For this review, take the finished solid that the model builds, in its own axes (mm). Give positions to 0.01 mm unless a question says otherwise; leave off trailing zeros. Order: outer loops, then holes, each group sorted by start corner. A loop starts at its lowest first (then second) coordinate and runs counter-clockwise, first axis right, second up.
Item 1: Consider section A-A (x = 0). Give the boundary of the cut face in (y, z).
Item 2: For probe 1 along X at (y, z) = (-40.5, -74); probe 2 along Y at (x, z) = (0, -71.5); probe 3 along Y at (x, z) = (-16.15, -70.75), list the stretches that pass through material, from the lowest coordinate up.
Item 3: Consider section C-C (x = 18.5). Give the boundary of the cut face in (y, z).
Item 4: For P1, Ø9.5, axis at x = 37.5, y = 0, coming from the +Z side; P2, Ø2.5, axis at x = 57, y = 24.5, coming from the +Z side, all flat-tipped, find the tip position at first contact; note any pin that passes through.
Item 5: Consider section D-D (x = 44). Give the boundary of the cut face in (y, z).
Item 6: Consider section B-B (x = 58.85). Give the boundary of the cut face in (y, z), plus the area to 3 significant figures.
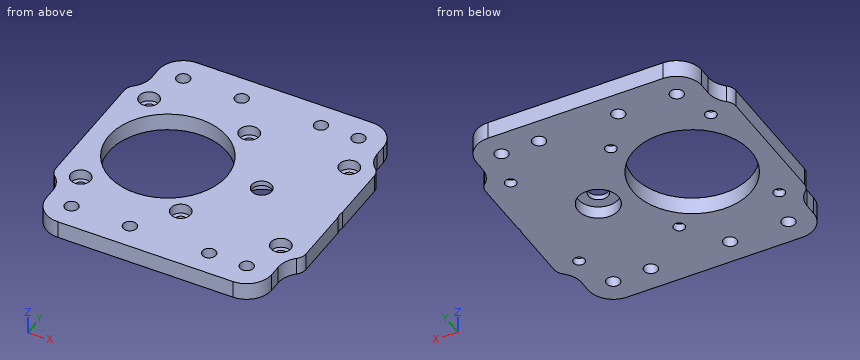
```python
from build123d import *

# Parameters (mm, degrees)
SKETCH2_R                      = 2.15
SKETCH2_R_2                    = 23.6
BOSS_EXTRUDE1_DEPTH            = 7
CUT_EXTRUDE1_START             = -7
SKETCH3_R                      = 8.1
SKETCH3_R_2                    = 23.6
CUT_EXTRUDE1_DEPTH             = 5
SKETCH4_R                      = 4
CUT_EXTRUDE2_DEPTH             = 5
SKETCH5_R                      = 6.365
CUT_EXTRUDE3_DEPTH             = 10
CBORE_FOR_M4_SHCS1_D           = 4.5
CBORE_FOR_M4_SHCS1_CBORE_D     = 8
CBORE_FOR_M4_SHCS1_CBORE_DEPTH = 4
SKETCH9_W                      = 90
SKETCH9_H                      = 20.85
SKETCH9_R                      = 2.7
BOSS_EXTRUDE3_DEPTH            = 7
FILLET2_R                      = 10
SKETCH10_W                     = 55
SKETCH10_H                     = 101.7
SKETCH10_R                     = 23.6
SKETCH10_R_2                   = 2.25
SKETCH10_R_3                   = 2.7
BOSS_EXTRUDE4_DEPTH            = 7


with BuildPart() as part:
    # Sketch2 → Boss-Extrude1 (new body)
    with BuildSketch(Plane.XY.offset(-75.526253649)):
        with BuildLine():
            Line((63.85, 30), (-26.15, 30))
            ThreePointArc((-26.15, 30), (-29.685533906, 28.535533906), (-31.15, 25))
            Line((-31.15, 25), (-31.15, -25))
            ThreePointArc((-31.15, -25), (-29.685533906, -28.535533906), (-26.15, -30))
            Line((-26.15, -30), (63.85, -30))
            ThreePointArc((63.85, -30), (67.385533906, -28.535533906), (68.85, -25))
            Line((68.85, -25), (68.85, 25))
            ThreePointArc((68.85, 25), (67.385533906, 28.535533906), (63.85, 30))
        make_face()
        with Locations((58.85, 25)):
            Circle(SKETCH2_R, mode=Mode.SUBTRACT)
        with Locations((18.85, 25)):
            Circle(SKETCH2_R, mode=Mode.SUBTRACT)
        with Locations((-21.15, 25)):
            Circle(SKETCH2_R, mode=Mode.SUBTRACT)
        with Locations((-21.15, -25)):
            Circle(SKETCH2_R, mode=Mode.SUBTRACT)
        with Locations((18.85, -25)):
            Circle(SKETCH2_R, mode=Mode.SUBTRACT)
        with Locations((58.85, -25)):
            Circle(SKETCH2_R, mode=Mode.SUBTRACT)
        Circle(SKETCH2_R_2, mode=Mode.SUBTRACT)
    extrude(amount=BOSS_EXTRUDE1_DEPTH)

    # Sketch3 → Cut-Extrude1 (cut)
    with BuildSketch(Plane.XY.offset(-68.526253649).offset(CUT_EXTRUDE1_START)):
        with Locations((37.5, 0)):
            Circle(SKETCH3_R)
        Circle(SKETCH3_R_2)
    extrude(amount=CUT_EXTRUDE1_DEPTH, mode=Mode.SUBTRACT)

    # Sketch4 → Cut-Extrude2 (cut)
    with BuildSketch(Plane(origin=(0, 0, -70.526253649), x_dir=(-1, 0, 0), z_dir=(0, 0, -1))):
        with Locations((-37.5, 0)):
            Circle(SKETCH4_R)
    extrude(amount=-CUT_EXTRUDE2_DEPTH, mode=Mode.SUBTRACT)

    # Sketch5 → Cut-Extrude3 (cut)
    with BuildSketch(Plane.XY.offset(-68.526253649)):
        with Locations((75, 0)):
            Circle(SKETCH5_R)
    extrude(amount=-CUT_EXTRUDE3_DEPTH, mode=Mode.SUBTRACT)

    # CBORE for M4 SHCS1 (through all)
    with Locations(Plane(origin=(-21.15, 25, -68.526253649), x_dir=(1, 0, 0), z_dir=(0, 0, 1))):
        with Locations((0, 0), (40, 0), (80, 0), (80, -50), (40, -50), (0, -50)):
            CounterBoreHole(CBORE_FOR_M4_SHCS1_D / 2, CBORE_FOR_M4_SHCS1_CBORE_D / 2, CBORE_FOR_M4_SHCS1_CBORE_DEPTH)

    # Sketch9 → Boss-Extrude3 (add)
    with BuildSketch(Plane.XY.offset(-68.526253649)):
        with Locations((18.85, 40.425)):
            Rectangle(SKETCH9_W, SKETCH9_H)
        with Locations((-16.15, 40.85)):
            Circle(SKETCH9_R, mode=Mode.SUBTRACT)
        with Locations((7.183333333, 40.85)):
            Circle(SKETCH9_R, mode=Mode.SUBTRACT)
        with Locations((53.85, 40.85)):
            Circle(SKETCH9_R, mode=Mode.SUBTRACT)
        with Locations((38.85, 40.85)):
            Circle(SKETCH9_R, mode=Mode.SUBTRACT)
        with Locations((18.85, -40.425)):
            Rectangle(SKETCH9_W, SKETCH9_H)
        with Locations((53.85, -40.85)):
            Circle(SKETCH9_R, mode=Mode.SUBTRACT)
        with Locations((7.183333333, -40.85)):
            Circle(SKETCH9_R, mode=Mode.SUBTRACT)
        with Locations((-16.15, -40.85)):
            Circle(SKETCH9_R, mode=Mode.SUBTRACT)
        with Locations((38.85, -40.85)):
            Circle(SKETCH9_R, mode=Mode.SUBTRACT)
    extrude(amount=-BOSS_EXTRUDE3_DEPTH)

    # Fillet2
    fillet2_edges = [part.edges().sort_by_distance(p)[0] for p in [
        (63.85, 50.85, -72.026253649),
        (-26.15, 50.85, -72.026253649),
        (63.85, -30, -72.026253649),
        (-26.15, -30, -72.026253649),
        (-26.15, 30, -72.026253649),
        (63.85, 30, -72.026253649),
        (-26.15, -50.85, -72.026253649),
        (63.85, -50.85, -72.026253649),
    ]]
    fillet(fillet2_edges, radius=FILLET2_R)


with BuildPart() as body_2:
    # Sketch10 → Boss-Extrude4 (new body)
    with BuildSketch(Plane.XY.offset(-68.526253649)):
        Rectangle(SKETCH10_W, SKETCH10_H)
        Circle(SKETCH10_R, mode=Mode.SUBTRACT)
        with Locations((-21.15, 25)):
            Circle(SKETCH10_R_2, mode=Mode.SUBTRACT)
        with Locations((18.85, 25)):
            Circle(SKETCH10_R_2, mode=Mode.SUBTRACT)
        with Locations((18.85, -25)):
            Circle(SKETCH10_R_2, mode=Mode.SUBTRACT)
        with Locations((-21.15, -25)):
            Circle(SKETCH10_R_2, mode=Mode.SUBTRACT)
        with Locations((-16.15, -40.85)):
            Circle(SKETCH10_R_3, mode=Mode.SUBTRACT)
        with Locations((7.183333333, -40.85)):
            Circle(SKETCH10_R_3, mode=Mode.SUBTRACT)
        with Locations((7.183333333, 40.85)):
            Circle(SKETCH10_R_3, mode=Mode.SUBTRACT)
        with Locations((-16.15, 40.85)):
            Circle(SKETCH10_R_3, mode=Mode.SUBTRACT)
    extrude(amount=BOSS_EXTRUDE4_DEPTH)


solid = part.part
```
Resolved:
1. outline: (-50.85, -75.53) - (-23.6, -75.53) - (-23.6, -68.53) - (-50.85, -68.53) - close; (23.6, -75.53) - (50.85, -75.53) - (50.85, -68.53) - (23.6, -68.53) - close
2. probe 1: x = -26.15 to -18.83, -13.47 to 4.51, 9.86 to 36.17, 41.53 to 51.17, 56.53 to 63.85
2. probe 2: y = -50.85 to -23.6, 23.6 to 50.85
2. probe 3: y = -50.85 to -43.55, -38.15 to -17.21, 17.21 to 38.15, 43.55 to 50.85
3. outline: (-50.85, -75.53) - (-27.22, -75.53) - (-27.22, -72.53) - (-28.98, -72.53) - (-28.98, -68.53) - (-50.85, -68.53) - close; (-22.78, -75.53) - (-14.65, -75.53) - (-14.65, -68.53) - (-21.02, -68.53) - (-21.02, -72.53) - (-22.78, -72.53) - close; (14.65, -75.53) - (22.78, -75.53) - (22.78, -72.53) - (21.02, -72.53) - (21.02, -68.53) - (14.65, -68.53) - close; (27.22, -75.53) - (50.85, -75.53) - (50.85, -68.53) - (28.98, -68.53) - (28.98, -72.53) - (27.22, -72.53) - close
4. P1: stops at z = -68.53
4. P2: stops at z = -72.53
5. outline: (-50.85, -75.53) - (-4.83, -75.53) - (-4.83, -70.53) - (4.83, -70.53) - (4.83, -75.53) - (50.85, -75.53) - (50.85, -68.53) - (-50.85, -68.53) - close
6. outline: (-49.51, -75.53) - (-27.25, -75.53) - (-27.25, -72.53) - (-29, -72.53) - (-29, -68.53) - (-49.51, -68.53) - close; (-22.75, -75.53) - (22.75, -75.53) - (22.75, -72.53) - (21, -72.53) - (21, -68.53) - (-21, -68.53) - (-21, -72.53) - (-22.75, -72.53) - close; (27.25, -75.53) - (49.51, -75.53) - (49.51, -68.53) - (29, -68.53) - (29, -72.53) - (27.25, -72.53) - close
6. area: 602 mm2
